Work out the finished part from the listing and answer in its coordinate system (mm). A direction names the side the tool comes from. Coordinates: 2 decimals unless noted, no trailing zeros. Loops run counter-clockwise (first coordinate to the right, second up) from the corner with the lowest first, then second, coordinate; pieces in that order, holes last. Notation, with made-up numbers: (28, 15.5) - (47, 15.5) arc R20 ccw to (47, 36.5) - close; hole circle Ø2 at (51.5, -13). An arc over 180 degrees is marked (long way). Write each question's results on one line, items separated by ' | '. Start each with the question number.
1. Find the intervals of material crossed by line 1 along Y through (x, z) = (-17, 21.59); line 2 along Z through (x, y) = (0, 18.1), in increasing order. Write a range as [from, to].
2. A cutting plane is placed at A-A on z = 21.59. Determine the outline of the cut face in (x, y) (3 decimals), then the cut area to 3 significant figures.
3. A cutting plane is placed at D-D on z = 6.5. Determine the outline of the cut face in (x, y) (3 decimals).
4. Each of these flat-tipped pins is pushed along its axis until it touches: P1, Ø2.5, axis at x = 0, z = 21.59, coming from the +Y side; P2, Ø3.5, axis at x = 0, z = 21.59, coming from the +Y side. Where does it stop, or does it pass through?
5. A cutting plane is placed at B-B on y = 0. Determine the outline of the cut face in (x, z) (3 decimals), then the cut area to 3 significant figures.
6. Which of the six approach directions +Z, -Z, +X, -X, +Y, -Y give full straight-line access (tool end or side, diameter ignored) to faces 4 (the flat face through (-19.05, 0, 19)), 5 (the flat face through (0, 0, 25.4))?
7. Determine the mould class of faces 1 (the cylindrical face through (13.93, -4.39, 12.52)), 2 (the cylindrical face through (-0.303, -16.824, 20.226)), 3 (the flat face through (0, 19.05, 19)) for opening direction Y: released by +Y, released by -Y, zero draft, split by the parting line, or undercut.
from build123d import *

# Parameters (mm, degrees)
F0_W     = 38.1
F0_H     = 38.1
F1_DEPTH = 38.1
F2_R     = 14.605
F3_DEPTH = 25.4
F5_D     = 2.794
F7_D     = 2.794


with BuildPart() as f1:
    # F0 (on Top) → F1 (new body)
    with BuildSketch(Plane.XY):
        Rectangle(F0_W, F0_H)
    extrude(amount=F1_DEPTH)

    # F2 (on face) → F3 (cut)
    with BuildSketch(Plane(origin=(0, 0, 0), x_dir=(1, 0, 0), z_dir=(0, 0, -1))):
        Circle(F2_R)
    extrude(amount=-F3_DEPTH, mode=Mode.SUBTRACT)

    # F5 (through all)
    with Locations(Plane(origin=(0, 19.05, 0), x_dir=(-1, 0, 0), z_dir=(0, 1, 0))):
        with Locations((0, 21.59)):
            Hole(F5_D / 2)

    # F7 (through all)
    with Locations(Plane.YZ.offset(19.05)):
        with Locations((0, 21.59)):
            Hole(F7_D / 2)


solid = f1.part
Values:
1) line 1: [-19.05, -1.4], [1.4, 19.05] | line 2: [0, 20.19], [22.99, 38.1]
2) outline: (-19.05, -19.05) - (-1.397, -19.05) - (-1.397, -14.538) arc R14.605 cw to (-14.538, -1.397) - (-19.05, -1.397) - close; (-19.05, 1.397) - (-14.538, 1.397) arc R14.605 cw to (-1.397, 14.538) - (-1.397, 19.05) - (-19.05, 19.05) - close; (1.397, -19.05) - (19.05, -19.05) - (19.05, -1.397) - (14.538, -1.397) arc R14.605 cw to (1.397, -14.538) - close; (1.397, 14.538) arc R14.605 cw to (14.538, 1.397) - (19.05, 1.397) - (19.05, 19.05) - (1.397, 19.05) - close | area: 732 mm^2
3) outline: (-19.05, -19.05) - (19.05, -19.05) - (19.05, 19.05) - (-19.05, 19.05) - close; hole circle Ø29.21 at (0, 0)
4) P1: through | P2: y = 19.05
5) outline: (-19.05, 0) - (-14.605, 0) - (-14.605, 20.193) - (-19.05, 20.193) - close; (-19.05, 22.987) - (-14.605, 22.987) - (-14.605, 25.4) - (14.605, 25.4) - (14.605, 22.987) - (19.05, 22.987) - (19.05, 38.1) - (-19.05, 38.1) - close; (14.605, 0) - (19.05, 0) - (19.05, 20.193) - (14.605, 20.193) - close | area: 685 mm^2
6) face 4: +Z, -Z, -X, +Y, -Y | face 5: -Z
7) face 1: undercut | face 2: zero draft | face 3: released by +Y
